```python
from build123d import *

# Parameters (mm, degrees)
SKETCH1_R           = 1.5
BOSS_EXTRUDE1_DEPTH = 3
SKETCH2_W           = 20
SKETCH2_H           = 50
BOSS_EXTRUDE2_DEPTH = 8


with BuildPart() as part:
    # Sketch1 → Boss-Extrude1 (new body)
    with BuildSketch(Plane(origin=(0, 0, 0), x_dir=(-1, 0, 0), z_dir=(0, 0, 1))):
        Polygon((50.75, 10.25), (50.75, 48.25), (50.75, 57.25), (-50.75, 57.25), (-50.75, -14.25), (-50.75, -41.25), (-50.75, -57.25), (-43.25, -57.25), (29.75, -57.25), (50.75, -57.25), (50.75, -46.75), (38.75, -46.75), (38.75, -34.75), (50.75, -34.75), (50.75, -29.75), (50.75, -20.75), (50.75, -11.75), (25.25, -11.75), (25.25, 4.25), (50.75, 4.25), align=None)
        with Locations(Location((-47, -53.5, 0), (0, 0, 180))):
            Circle(SKETCH1_R, mode=Mode.SUBTRACT)
        with Locations(Location((-47, 53.5, 0), (0, 0, 180))):
            Circle(SKETCH1_R, mode=Mode.SUBTRACT)
        with Locations(Location((47, 53.5, 0), (0, 0, 180))):
            Circle(SKETCH1_R, mode=Mode.SUBTRACT)
        with Locations(Location((47, -53.5, 0), (0, 0, 180))):
            Circle(SKETCH1_R, mode=Mode.SUBTRACT)
    extrude(amount=BOSS_EXTRUDE1_DEPTH)

    # Sketch2 → Boss-Extrude2 (add)
    with BuildSketch(Plane(origin=(0, 0, 0), x_dir=(-1, 0, 0), z_dir=(0, 0, -1))):
        with Locations((-7.252332969, 0)):
            Rectangle(SKETCH2_W, SKETCH2_H)
    extrude(amount=-BOSS_EXTRUDE2_DEPTH)


solid = part.part
```
For this review, take the finished solid that the model builds, in its own axes (mm). A direction names the side the tool comes from. Give positions to 0.01 mm unless a question says otherwise; leave off trailing zeros. Order: outer loops, then holes, each group sorted by start corner. A loop starts at its lowest first (then second) coordinate and runs counter-clockwise, first axis right, second up.
1) Take a section at B-B (y = -53.5). Give the boundary of the cut face in (x, z), then the cut area to 4 significant figures.
2) The part is to be moulded in two halves that separate along X. For faces 1 (the face through (-48.2, 52.6, 1.5)), 2 (the face through (-50.75, -30, 1)), 3 (the face through (7, -25, 5)), say which applies: released by +X, released by -X, zero draft, split by the parting line, or undercut.
3) For faces 4 (the face through (7, 25, 5)), 5 (the face through (-45, 34.75, 1)), 6 (the face through (17.252, 0, 5)), list the 3-axis set-ups (+Z, -Z, +X, -X, +Y, -Y) from which the entire face can be reached by the end or side of a thin tool; tool diameter is ignored.
4) Take a section at A-A (x = -47). Give the boundary of the cut face in (y, z), then the cut area to 4 significant figures.
5) Insertion check: pin 1 (1 mm diameter, centred on y = 0, z = 1, fed in from -X); pin 2 (2.5 mm diameter, centred on y = 5, z = 4.5, fed in from -X); pin 3 (3.5 mm diameter, centred on y = 42.5, z = 1.5, fed in from -X). Each pin has a flat end and moves straight along its axis. Give the tip position at first contact, or say it passes through.
6) Take a section at D-D (y = 2). Give the boundary of the cut face in (x, z).
7) Take a section at C-C (x = -26.5). Give the boundary of the cut face in (y, z).
8) Wall thickness on line 1 (Y direction, x = -47, z = 2); line 2 (Y direction, x = 47, z = 2.3); line 3 (X direction, y = 41, z = 2.75): over which ranges is each line inside the solid? List them lowest first.
Derived:
1. outline: (-50.75, 0) - (-48.5, 0) - (-48.5, 3) - (-50.75, 3) - close; (-45.5, 0) - (45.5, 0) - (45.5, 3) - (-45.5, 3) - close; (48.5, 0) - (50.75, 0) - (50.75, 3) - (48.5, 3) - close
1. area: 286.5 mm2
2. face 1: undercut
2. face 2: released by -X
2. face 3: zero draft
3. face 4: +Z, +X, -X, +Y
3. face 5: +Z, -Z, -X
3. face 6: +Z, +X, +Y, -Y
4. outline: (-57.25, 0) - (-55, 0) - (-55, 3) - (-57.25, 3) - close; (-52, 0) - (-4.25, 0) - (-4.25, 3) - (-52, 3) - close; (11.75, 0) - (34.75, 0) - (34.75, 3) - (11.75, 3) - close; (46.75, 0) - (52, 0) - (52, 3) - (46.75, 3) - close; (55, 0) - (57.25, 0) - (57.25, 3) - (55, 3) - close
4. area: 241.5 mm2
5. pin 1: stops at x = -25.25
5. pin 2: stops at x = -2.75
5. pin 3: stops at x = -38.75
6. outline: (-25.25, 0) - (50.75, 0) - (50.75, 3) - (17.25, 3) - (17.25, 8) - (-2.75, 8) - (-2.75, 3) - (-25.25, 3) - close
7. outline: (-57.25, 0) - (-4.25, 0) - (-4.25, 3) - (-57.25, 3) - close; (11.75, 0) - (57.25, 0) - (57.25, 3) - (11.75, 3) - close
8. line 1: y = -57.25 to -55, -52 to -4.25, 11.75 to 34.75, 46.75 to 52, 55 to 57.25
8. line 2: y = -57.25 to -55, -52 to 52, 55 to 57.25
8. line 3: x = -38.75 to 50.75
